from build123d import *

# Parameters (mm, degrees)
SKIZZE1_R                       = 32.4
SKIZZE1_R_2                     = 1.8
AUFSATZ_LINEAR_AUSTRAGEN1_DEPTH = 3
SCHNITT_LINEAR_AUSTRAGEN1_DEPTH = 46.918623673
AUFSATZ_LINEAR_START            = 18
SKIZZE4_R                       = 0.85
SKIZZE4_W                       = 4.8
SKIZZE4_H                       = 12.19937625
AUFSATZ_LINEAR_AUSTRAGEN2_DEPTH = 18
SKIZZE5_W                       = 2
SKIZZE5_H                       = 5
SCHNITT_LINEAR_AUSTRAGEN2_DEPTH = 18
SKIZZE6_W                       = 10
SKIZZE6_H                       = 5
SCHNITT_LINEAR_AUSTRAGEN3_DEPTH = 18
FL_CHE_VERSCHIEBEN1_BY          = 1.5
SKIZZE8_R                       = 35
SKIZZE8_R_2                     = 32.4
AUFSATZ_LINEAR_AUSTRAGEN3_DEPTH = 3
SKIZZE9_R                       = 1.8
SKIZZE9_R_2                     = 1.6
AUFSATZ_LINEAR_AUSTRAGEN4_DEPTH = 4.5
FL_CHE_VERSCHIEBEN2_OUTLINE_R   = 35
FL_CHE_VERSCHIEBEN2_OUTLINE_R_2 = 1.6
FL_CHE_VERSCHIEBEN2_OUTLINE_W   = 4.8
FL_CHE_VERSCHIEBEN2_OUTLINE_H   = 12.19937625
FL_CHE_VERSCHIEBEN2_DEPTH       = 1.5
SKIZZE10_R                      = 36.675991258
SKIZZE10_R_2                    = 32.4
SCHNITT_LINEAR_AUSTRAGEN4_DEPTH = 1.5
FASE1_SIZE                      = 0.5


# Read off the part's stored shape, not the designer's step: Fläche verschieben2
with BuildPart() as part:
    # Skizze1 → Aufsatz-Linear austragen1 (new body)
    with BuildSketch(Plane.XY):
        Circle(SKIZZE1_R)
        with Locations((-20, -20)):
            Circle(SKIZZE1_R_2, mode=Mode.SUBTRACT)
        with Locations((20, -20)):
            Circle(SKIZZE1_R_2, mode=Mode.SUBTRACT)
        with Locations((20, 20)):
            Circle(SKIZZE1_R_2, mode=Mode.SUBTRACT)
        with Locations((-20, 20)):
            Circle(SKIZZE1_R_2, mode=Mode.SUBTRACT)
    extrude(amount=-AUFSATZ_LINEAR_AUSTRAGEN1_DEPTH)

    # Skizze2 → Schnitt-Linear austragen1 (cut, through all)
    with BuildSketch(Plane.XY):
        with BuildLine():
            ThreePointArc((5, 5.590169944), (0, 7.5), (-5, 5.590169944))
            ThreePointArc((-5, 5.590169944), (-5.511799249, 5.289873919), (-6.1, 5.211540978))
            ThreePointArc((-6.1, 5.211540978), (-6.859313681, 5.478740636), (-7.371163001, 6.1))
            ThreePointArc((-7.371163001, 6.1), (-7.466484857, 7.023516737), (-7, 7.826237921))
            ThreePointArc((-7, 7.826237921), (0, 10.5), (7, 7.826237921))
            ThreePointArc((7, 7.826237921), (7.118033989, 5.708203932), (5, 5.590169944))
        make_face()
        with BuildLine():
            ThreePointArc((-7, -7.826237921), (0, -10.5), (7, -7.826237921))
            ThreePointArc((7, -7.826237921), (7.118033989, -5.708203932), (5, -5.590169944))
            ThreePointArc((5, -5.590169944), (0, -7.5), (-5, -5.590169944))
            ThreePointArc((-5, -5.590169944), (-5.511799249, -5.289873919), (-6.1, -5.211540978))
            ThreePointArc((-6.1, -5.211540978), (-6.859313681, -5.478740636), (-7.371163001, -6.1))
            ThreePointArc((-7.371163001, -6.1), (-7.466484857, -7.023516737), (-7, -7.826237921))
        make_face()
    extrude(amount=-SCHNITT_LINEAR_AUSTRAGEN1_DEPTH, mode=Mode.SUBTRACT)

    # Skizze4 → Aufsatz-Linear austragen2 (add)
    # profile 1 of 2: a face of its own
    with BuildSketch(Plane.XY.offset(AUFSATZ_LINEAR_START)):
        with BuildLine():
            Line((-10.9, 6.1), (-10.9, -6.1))
            Line((-10.9, -6.1), (-7.371163001, -6.1))
            ThreePointArc((-7.371163001, -6.1), (-6.859313681, -5.478740636), (-6.1, -5.211540978))
            Line((-6.1, -5.211540978), (-6.1, 0.782623792))
            Line((-6.1, 0.782623792), (-6.1, 5.211540978))
            ThreePointArc((-6.1, 5.211540978), (-6.859313681, 5.478740636), (-7.371163001, 6.1))
            Line((-7.371163001, 6.1), (-10.9, 6.1))
        make_face()
        with Locations((-8.5, 0)):
            Circle(SKIZZE4_R, mode=Mode.SUBTRACT)
    # profile 2 of 2: a face of its own
    with BuildSketch(Plane.XY.offset(AUFSATZ_LINEAR_START)):
        with Locations((19.25, 0)):
            Rectangle(SKIZZE4_W, SKIZZE4_H)
        with Locations((19.25, 0)):
            Circle(SKIZZE4_R, mode=Mode.SUBTRACT)
    extrude(amount=-AUFSATZ_LINEAR_AUSTRAGEN2_DEPTH)

    # Skizze5 → Schnitt-Linear austragen2 (cut)
    with BuildSketch(Plane.XY.offset(18)):
        with Locations((-6.1, 0)):
            Rectangle(SKIZZE5_W, SKIZZE5_H)
    extrude(amount=-SCHNITT_LINEAR_AUSTRAGEN2_DEPTH, mode=Mode.SUBTRACT)

    # Skizze6 → Schnitt-Linear austragen3 (cut)
    with BuildSketch(Plane.ZY.offset(10.9)):
        with Locations((5, 0)):
            Rectangle(SKIZZE6_W, SKIZZE6_H)
    extrude(amount=-SCHNITT_LINEAR_AUSTRAGEN3_DEPTH, mode=Mode.SUBTRACT)

    # Fläche verschieben1: a face moved outward by 1.5
    extrude(part.faces().sort_by_distance((0, 0, -3))[0], amount=FL_CHE_VERSCHIEBEN1_BY, dir=(0, 0, -1))

    # Skizze8 → Aufsatz-Linear austragen3 (add)
    with BuildSketch(Plane.XY):
        Circle(SKIZZE8_R)
        Circle(SKIZZE8_R_2, mode=Mode.SUBTRACT)
    extrude(amount=-AUFSATZ_LINEAR_AUSTRAGEN3_DEPTH)

    # Skizze9 → Aufsatz-Linear austragen4 (add)
    # profile 1 of 4: a face of its own
    with BuildSketch(Plane.XY):
        with Locations((-20, 20)):
            Circle(SKIZZE9_R)
        with Locations((-20, 20)):
            Circle(SKIZZE9_R_2, mode=Mode.SUBTRACT)
    # profile 2 of 4: a face of its own
    with BuildSketch(Plane.XY):
        with Locations((20, 20)):
            Circle(SKIZZE9_R)
        with Locations((20, 20)):
            Circle(SKIZZE9_R_2, mode=Mode.SUBTRACT)
    # profile 3 of 4: a face of its own
    with BuildSketch(Plane.XY):
        with Locations((20, -20)):
            Circle(SKIZZE9_R)
        with Locations((20, -20)):
            Circle(SKIZZE9_R_2, mode=Mode.SUBTRACT)
    # profile 4 of 4: a face of its own
    with BuildSketch(Plane.XY):
        with Locations((-20, -20)):
            Circle(SKIZZE9_R)
        with Locations((-20, -20)):
            Circle(SKIZZE9_R_2, mode=Mode.SUBTRACT)
    extrude(amount=-AUFSATZ_LINEAR_AUSTRAGEN4_DEPTH)

    # Fläche verschieben2 outline → Fläche verschieben2 (add)
    with BuildSketch(Plane.XY):
        Circle(FL_CHE_VERSCHIEBEN2_OUTLINE_R)
        with Locations((-20, -20)):
            Circle(FL_CHE_VERSCHIEBEN2_OUTLINE_R_2, mode=Mode.SUBTRACT)
        with BuildLine():
            ThreePointArc((7, -7.826237921), (0, -10.5), (-7, -7.826237921))
            ThreePointArc((-7, -7.826237921), (-7.466484857, -7.023516737), (-7.371163002, -6.1))
            Line((-7.371163002, -6.1), (-10.9, -6.1))
            Line((-10.9, -6.1), (-10.9, -2.5))
            Line((-10.9, -2.5), (-6.1, -2.5))
            Line((-6.1, -2.5), (-6.1, -5.211540977))
            ThreePointArc((-6.1, -5.211540977), (-5.511799249, -5.289873919), (-5, -5.590169944))
            ThreePointArc((-5, -5.590169944), (0, -7.5), (5, -5.590169944))
            ThreePointArc((5, -5.590169944), (7.118033989, -5.708203932), (7, -7.826237921))
        make_face(mode=Mode.SUBTRACT)
        with Locations((20, -20)):
            Circle(FL_CHE_VERSCHIEBEN2_OUTLINE_R_2, mode=Mode.SUBTRACT)
        with BuildLine():
            Line((-6.1, 2.5), (-10.9, 2.5))
            Line((-10.9, 2.5), (-10.9, 6.1))
            Line((-10.9, 6.1), (-7.371163002, 6.1))
            ThreePointArc((-7.371163002, 6.1), (-7.466484857, 7.023516737), (-7, 7.826237921))
            ThreePointArc((-7, 7.826237921), (0, 10.5), (7, 7.826237921))
            ThreePointArc((7, 7.826237921), (7.118033989, 5.708203932), (5, 5.590169944))
            ThreePointArc((5, 5.590169944), (0, 7.5), (-5, 5.590169944))
            ThreePointArc((-5, 5.590169944), (-5.511799249, 5.289873919), (-6.1, 5.211540977))
            Line((-6.1, 5.211540977), (-6.1, 2.5))
        make_face(mode=Mode.SUBTRACT)
        with Locations((-20, 20)):
            Circle(FL_CHE_VERSCHIEBEN2_OUTLINE_R_2, mode=Mode.SUBTRACT)
        with Locations((19.25, 0)):
            Rectangle(FL_CHE_VERSCHIEBEN2_OUTLINE_W, FL_CHE_VERSCHIEBEN2_OUTLINE_H, mode=Mode.SUBTRACT)
        with Locations((20, 20)):
            Circle(FL_CHE_VERSCHIEBEN2_OUTLINE_R_2, mode=Mode.SUBTRACT)
    extrude(amount=FL_CHE_VERSCHIEBEN2_DEPTH)

    # Skizze10 → Schnitt-Linear austragen4 (cut)
    with BuildSketch(Plane.XY.offset(1.5)):
        Circle(SKIZZE10_R)
        Circle(SKIZZE10_R_2, mode=Mode.SUBTRACT)
    extrude(amount=-SCHNITT_LINEAR_AUSTRAGEN4_DEPTH, mode=Mode.SUBTRACT)

    # Fase1
    fase1_edges = [part.edges().sort_by_distance(p)[0] for p in [
        (-35, 0, -3),
        (-35, 0, 0),
    ]]
    chamfer(fase1_edges, length=FASE1_SIZE)


solid = part.part
Source: CAD feature listing. Evaluate the final solid. Frame: model axes, mm. A direction names the side the tool comes from. Give positions to 0.01 mm unless a question says otherwise; leave off trailing zeros. Write each loop counter-clockwise with the first axis right and the second up, starting at its lowest first coordinate (ties: lowest second). Pieces come first, ordered by that corner, then holes. Notation, with made-up numbers: (-5, -21.75) -> (23, -21.75) arc R20 cw to (23, -1.75) -> close; hole circle Ø3 at (86, 58.5). An arc over 180 degrees is marked (long way). Return JSON: item names as keys, results as strings. Group by question number.
1. Mould query, pull axis X, two halves, no side actions, for faces 1 (the face through (16.85, 0, 10)), 2 (the face through (19, 6.1, 10)), 3 (the face through (21.65, 0, 10)). Classes: +X half, -X half, draft (parallel to the pull), parting line (faces both ways), or undercut.
2. Section B-B, the plane z = 3. Output: boundary loops of the cut face in (x, y).
3. Section A-A, the plane z = 16. Output: boundary loops of the cut face in (x, y).
4. Section C-C, the plane x = 19.25. Count the separate pieces of the cut face and the enclosed holes in it, then the cut area to 3 significant figures.
5. Pin query (flat end, axial travel): pin 1 Ø1.4 at (x, z) = (19, 8.5) entering from -Y; pin 2 Ø1.4 at (x, y) = (-8.5, 0) entering from +Z; pin 3 Ø0.8 at (y, z) = (-4, 9.5) entering from +X. Return the tip coordinate at first contact, or that it passes through.
6. Material intervals for line 1 (Y direction, x = 19.25, z = 5.5); line 2 (Y direction, x = 20, z = -0.6); line 3 (Z direction, x = -20, y = 25), sorted ascending. Write a range as from..to.
7. Access query for faces 4 (the face through (0.1, -10.5, -1.5)), 5 (the face through (-8, -2.5, 8)), 6 (the face through (-7.02, -31.63, 0.76)), 7 (the face through (-7.02, -31.63, -3.74)). Directions: +Z, -Z, +X, -X, +Y, -Y. A direction counts if a zero-diameter tool reaches every point of the face in a straight line with its end or side. Return the directions, or none.
Determined:
{
 "1": {"face 1": "undercut", "face 2": "draft", "face 3": "+X half"},
 "2": {"outline": "(-10.9, -6.1) -> (-7.37, -6.1) arc R1.5 cw to (-6.1, -5.21) -> (-6.1, -2.5) -> (-10.9, -2.5) -> close; (-10.9, 2.5) -> (-6.1, 2.5) -> (-6.1, 5.21) arc R1.5 cw to (-7.37, 6.1) -> (-10.9, 6.1) -> close; (16.85, -6.1) -> (21.65, -6.1) -> (21.65, 6.1) -> (16.85, 6.1) -> close; hole circle Ø1.7 at (19.25, 0)"},
 "3": {"outline": "(-10.9, -6.1) -> (-7.37, -6.1) arc R1.5 cw to (-6.1, -5.21) -> (-6.1, -2.5) -> (-7.1, -2.5) -> (-7.1, 2.5) -> (-6.1, 2.5) -> (-6.1, 5.21) arc R1.5 cw to (-7.37, 6.1) -> (-10.9, 6.1) -> close; (16.85, -6.1) -> (21.65, -6.1) -> (21.65, 6.1) -> (16.85, 6.1) -> close; hole circle Ø1.7 at (-8.5, 0); hole circle Ø1.7 at (19.25, 0)"},
 "4": {"separate pieces": "3", "enclosed holes": "0", "area": "468 mm2"},
 "5": {"pin 1": "stops at y = -6.1", "pin 2": "stops at z = 1.5", "pin 3": "stops at x = 21.65"},
 "6": {"line 1": "y = -6.1..-0.85, 0.85..6.1", "line 2": "y = -28.72..-21.6, -18.4..18.4, 21.6..28.72", "line 3": "z = -4.5..1.5"},
 "7": {"face 4": "+Z, -Z", "face 5": "none", "face 6": "+Z", "face 7": "-Z"}
}
